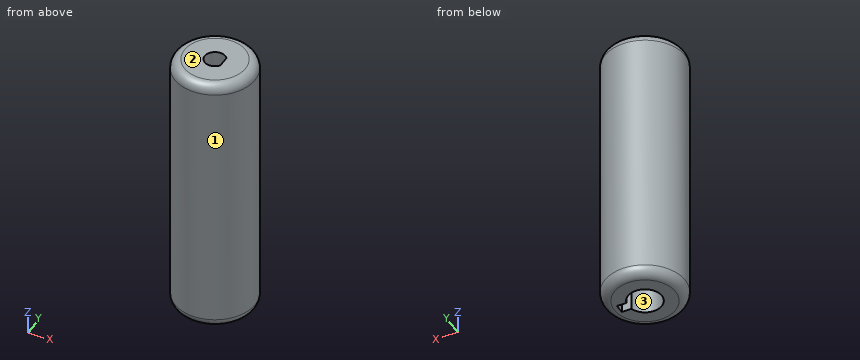
from build123d import *

# Parameters (mm, degrees)
F0_R     = 12.5
F1_DEPTH = 85
F2_DEPTH = 25
F4_DEPTH = 25
F5_R     = 3


with BuildPart() as f1:
    # F0 (on Top) → F1 (new body)
    with BuildSketch(Plane.XY):
        Circle(F0_R)
        with BuildLine():
            ThreePointArc((5.031153, -1.5), (-5.25, 0), (5.031153, 1.5))
            Line((5.031153, 1.5), (8.031153, 1.5))
            Line((8.031153, 1.5), (8.031153, -1.5))
            Line((8.031153, -1.5), (5.031153, -1.5))
        make_face(mode=Mode.SUBTRACT)
        with BuildLine():
            Line((5.031153, -1.5), (5.031153, 1.5))
            ThreePointArc((5.031153, 1.5), (-5.25, 0), (5.031153, -1.5))
        make_face()
        with BuildLine():
            ThreePointArc((5.031153, 1.5), (5.195, 0.75794), (5.25, 0))
            ThreePointArc((5.25, 0), (5.195, -0.75794), (5.031153, -1.5))
            Line((5.031153, -1.5), (8.031153, -1.5))
            Line((8.031153, -1.5), (8.031153, 1.5))
            Line((8.031153, 1.5), (5.031153, 1.5))
        make_face()
        with BuildLine():
            ThreePointArc((5.031153, -1.5), (5.195, -0.75794), (5.25, 0))
            ThreePointArc((5.25, 0), (5.195, 0.75794), (5.031153, 1.5))
            Line((5.031153, 1.5), (5.031153, -1.5))
        make_face()
    extrude(amount=F1_DEPTH)

    # F0 (on Top) → F2 (cut)
    with BuildSketch(Plane.XY):
        with BuildLine():
            Line((5.031153, -1.5), (5.031153, 1.5))
            ThreePointArc((5.031153, 1.5), (-5.25, 0), (5.031153, -1.5))
        make_face()
        with BuildLine():
            ThreePointArc((5.031153, -1.5), (5.195, -0.75794), (5.25, 0))
            ThreePointArc((5.25, 0), (5.195, 0.75794), (5.031153, 1.5))
            Line((5.031153, 1.5), (5.031153, -1.5))
        make_face()
        with BuildLine():
            ThreePointArc((5.031153, 1.5), (5.195, 0.75794), (5.25, 0))
            ThreePointArc((5.25, 0), (5.195, -0.75794), (5.031153, -1.5))
            Line((5.031153, -1.5), (8.031153, -1.5))
            Line((8.031153, -1.5), (8.031153, 1.5))
            Line((8.031153, 1.5), (5.031153, 1.5))
        make_face()
    extrude(amount=F2_DEPTH, mode=Mode.SUBTRACT)

    # F3 (on face) → F4 (cut)
    with BuildSketch(Plane.XY.offset(85)):
        with BuildLine():
            Line((2.625, -1.873499), (2.625, 1.873499))
            ThreePointArc((2.625, 1.873499), (-3.225, 0), (2.625, -1.873499))
        make_face()
    extrude(amount=-F4_DEPTH, mode=Mode.SUBTRACT)

    # F5
    f5_edges = [f1.edges().sort_by_distance(p)[0] for p in [
        (-12.5, 0, 85),
        (-12.5, 0, 0),
    ]]
    fillet(f5_edges, radius=F5_R)


solid = f1.part
The model under review builds one solid part; all positions refer to its coordinate system, in mm. Face numbers are marked on the shaded views. Coordinates: 2 decimals unless noted, no trailing zeros. Write each loop counter-clockwise with the first axis right and the second up, starting at its lowest first coordinate (ties: lowest second). Pieces come first, ordered by that corner, then holes. Notation, with made-up numbers: (58.5, 62) - (79.5, 62) arc R17 ccw to (79.5, 83) - close; hole circle Ø9 at (79.5, 49.5). An arc over 180 degrees is marked (long way). Answer as CSV lines item,"result".
(1) We need section D-D (z = 56). Give the boundary of the cut face in (x, y).
Data:
outline,"circle Ø25 at (0, 0)"
(2) We need section C-C (y = 0). Give the boundary of the cut face in (x, z) (3 decimals).
Data:
outline,"(-12.5, 3) arc R3 ccw to (-9.5, 0) - (-5.25, 0) - (-5.25, 25) - (8.031, 25) - (8.031, 0) - (9.5, 0) arc R3 ccw to (12.5, 3) - (12.5, 82) arc R3 ccw to (9.5, 85) - (2.625, 85) - (2.625, 60) - (-3.225, 60) - (-3.225, 85) - (-9.5, 85) arc R3 ccw to (-12.5, 82) - close"
(3) For line 1 along Y through (x, z) = (0, 70) (3 decimals); line 2 along Y through (x, z) = (0, 19.5); line 3 along X through (y, z) = (-0.5, 61.5) (3 decimals), list the stretches that pass through material, from the lowest coordinate up. Write a range as [from, to].
Data:
line 1,"y = [-12.5, -3.225], [3.225, 12.5]"
line 2,"y = [-12.5, -5.25], [5.25, 12.5]"
line 3,"x = [-12.49, -3.186], [2.625, 12.49]"
(4) Mouldability with a two-part tool opening along X and no side actions: class the marked faces 1, 2 and 3 as pulls with the +X half, pulls with the -X half, needs draft (parallel to the pull), parting line crosses it, or undercut.
Data:
face 1,"parting line crosses it"
face 2,"needs draft"
face 3,"undercut"
(5) We need section A-A (z = 19). Give the boundary of the cut face in (x, y).
Data:
outline,"circle Ø25 at (0, 0); hole (5.03, -1.5) - (8.03, -1.5) - (8.03, 1.5) - (5.03, 1.5) arc R5.25 ccw (long way) to start"
(6) Clearance check with flat-ended pins moving along their axes: pin 1 Ø3 at (y, z) = (3.5, 21) entering from +X; pin 2 Ø8.5 at (x, y) = (0, 0) entering from -Z; pin 3 Ø1.5 at (x, z) = (-9.5, 76.5) entering from -Y. State where each tip first meets the part, or that it passes through.
Data:
pin 1,"stops at x = 12.34"
pin 2,"stops at z = 25"
pin 3,"stops at y = -8.93"
(7) We need section B-B (x = 0). Give the boundary of the cut face in (y, z) (3 decimals).
Data:
outline,"(-12.5, 3) arc R3 ccw to (-9.5, 0) - (-5.25, 0) - (-5.25, 25) - (5.25, 25) - (5.25, 0) - (9.5, 0) arc R3 ccw to (12.5, 3) - (12.5, 82) arc R3 ccw to (9.5, 85) - (3.225, 85) - (3.225, 60) - (-3.225, 60) - (-3.225, 85) - (-9.5, 85) arc R3 ccw to (-12.5, 82) - close"
